Part model, mm, in its own coordinate system. A direction names the side the tool comes from. Round coordinates to 2 decimals unless told otherwise and drop trailing zeros. Loops run counter-clockwise (first coordinate to the right, second up) from the corner with the lowest first, then second, coordinate; pieces in that order, holes last.
(1) Tool access for faces 4 (the face through (21.977, 25.266, 252.144)), 5 (the face through (0, 0, 252)): list every direction of +Z, -Z, +X, -X, +Y, -Y with a clear straight run to the whole face (end or side of a thin tool).
(2) Flat gauge pins, fed straight in: pin 1 (6 mm diameter, centred on x = 4.5, y = 12.5, fed in from +Z); pin 2 (1.5 mm diameter, centred on y = 13, z = 176.5, fed in from +X); pin 3 (4 mm diameter, centred on y = -13.5, z = 102, fed in from -X); pin 4 (5 mm diameter, centred on x = 25, y = 20.5, fed in from +Z). Where does each tip first touch, or does it go through?
(3) Cut at A-A on x = 15.5. List the corners of the cut face in (y, z), then the cut area to 3 significant figures.
(4) Probe probe 1 along Y at (x, z) = (9.5, 61.5); probe 2 along X at (y, z) = (6.5, 422.5); probe 3 along Z at (x, y) = (13.5, 29). List the from-to ranges inside material, lowest first.
(5) Cut at B-B on z = 349. List the corners of the cut face in (x, y), then the cut area to 3 significant figures.
(6) Mould opens along Y. For faces 1 (the face through (21.977, -25.266, 252.144)), 2 (the face through (18, -32.5, 252)), 3 (the face through (18, 32.5, 252)) say: +Y half, -Y half, draft (parallel to the pull), parting line (faces both ways), or undercut.
(7) Cut at C-C on y = -11.5. List the corners of the cut face in (x, z), then the cut area to 3 significant figures.
Autodesk Inventor part; units mm, degrees
ref_plane "Начальная плоскость" through (0, 0, 32.5001) normal (0, 0, 1) x (1, 0, 0)
ref_plane "Конечная плоскость" through (0, 0, 478.0035) normal (0, 0, 1) x (1, 0, 0)
ref_plane "РабПлоскость8" through (169.2997, 3.5, 32.958) normal (0.0027, 0, -1) x (-1, 0, -0.0027)
ref_plane "Начальная плоскость" through (0, 0, 32.5001) normal (0, 0, 1) x (1, 0, 0)
ref_plane "Конечная плоскость" through (0, 0, 478.0035) normal (0, 0, 1) x (1, 0, 0)
sketch "Эскиз" plane through (0, 0, 0) normal (0, 0, 1) x (1, 0, 0)
  line L0 (36, -32.5) -> (0, -32.5)
  line L1 (36, -32.5) -> (36, -28.696)
  line L2 (33.6994, -26.2039) -> (9.9215, -24.3017)
  line L3 (4.4, -18.3208) -> (4.4, 18.3208)
  line L4 (33.6994, 26.2039) -> (9.9215, 24.3017)
  line L5 (36, 28.696) -> (36, 32.5)
  line L6 (0, 32.5) -> (36, 32.5)
  line L7 (0, -32.5) -> (0, 32.5)
  arc A0 (4.4, -18.3208) -> (9.9215, -24.3017) centre (10.4, -18.3208) ccw
  arc A1 (9.9215, 24.3017) -> (4.4, 18.3208) centre (10.4, 18.3208) ccw
  arc A2 (36, -28.696) -> (33.6994, -26.2039) centre (33.5, -28.696) ccw
  arc A3 (33.6994, 26.2039) -> (36, 28.696) centre (33.5, 28.696) ccw
  line L8 (0, 45.5) -> (0, -45.5) construction
  line L9 (-7.2974, 0) -> (43.7847, 0) construction
  point P0 (36, -26.388)
  point P1 (4.4, -23.86)
  point P2 (4.4, 23.86)
  point P3 (36, 26.388)
  dimension "d3" = 36
  dimension "d5" = 4.4
  dimension "d7" = 65
  dimension "d9" = 8.64
  dimension "d11" = 8.64
  dimension "d13" = 6.112
  dimension "d15" = 6.112
  dimension "d22" = 6
  dimension "d23" = 2.5
  dimension "d24" = 32.5
  dimension "d25" = 0
extrude "Тело" add sketch "Эскиз" along normal up to surface (445.5034 mm away) from surface at 32.5001
sketch "Sketch3" plane through (0, 0, 0) normal (0, 0, 1) x (1, 0, 0)
  line L0 (0, 0) -> (10, 0)
ref_plane "Work Plane7" through (0, 0, 0) normal (0, -1, 0) x (1, 0, 0)
sketch "Sketch4" plane through (0, 0, 0) normal (0, -1, 0) x (1, 0, 0)
  line L0 (-2, 32.5001) -> (12, 32.5001)
  line L1 (-2, 478.0035) -> (12, 478.0035)
  dimension "d29" = 445.5034
ref_plane "РабПлоскость8" through (169.2997, 3.5, 32.958) normal (0.0027, 0, -1) x (-1, 0, -0.0027)
split "Разделение1" plane through (169.2997, 3.5, 32.958) removes the side toward (0.0027, 0, -1)
ref_plane "РабПлоскость9" through (164.2926, -32.5, 478.3501) normal (-0.0027, 0, 1) x (1, 0, 0.0027)
split "Разделение2" plane through (164.2926, -32.5, 478.3501) removes the side toward (-0.0027, 0, 1)
equation "\"d3\" = b"
equation "\"d7\" = ParH"
equation "\"d22\" = R"
equation "\"d23\" = R1"
equation "\"d24\" = 0.5 * d7"
equation "\"d16\" = G_L"
equation "\"R1\" = 2.5"
equation "\"R\" = 6"
equation "\"t1\" = 4.4"
equation "\"t2\" = 7.2"
equation "\"ParH\" = 65"
equation "\"b\" = 36"
equation "\"msp_x1\" = 0.04 * b"
equation "\"msp_x2\" = -0.08 * t1 + 0.04 * b"
equation "\"G_L\" = d29"
equation "\"ex\" = 0"
equation "\"G_OFFSET_START\" = -32.50012"
equation "\"G_OFFSET_END\" = -35.90288"
equation "\"d26\" = -G_OFFSET_START"
equation "\"d27\" = G_OFFSET_END + B_L"
equation "\"B_L\" = 513.90637"
properties part number "Швеллер 6.5U-445,5 ГОСТ 8240-97" material "Сталь, мягкая"
Final values:
1. face 4: +Z, -Z, +X
1. face 5: +Z, -Z, -X, +Y, -Y
2. pin 1: stops at z = 477.92
2. pin 2: stops at x = 4.4
2. pin 3: stops at x = 0
2. pin 4: passes through
3. outline: (-32.5, 32.54) - (-24.75, 32.54) - (-24.75, 477.95) - (-32.5, 477.95) - close; (24.75, 32.54) - (32.5, 32.54) - (32.5, 477.95) - (24.75, 477.95) - close
3. area: 6,910 mm2
4. probe 1: y = -32.5 to -24.25, 24.25 to 32.5
4. probe 2: x = 0 to 4.4
4. probe 3: z = 32.54 to 477.94
5. outline: (0, -32.5) - (36, -32.5) - (36, -28.7) arc R2.5 ccw to (33.7, -26.2) - (9.92, -24.3) arc R6 cw to (4.4, -18.32) - (4.4, 18.32) arc R6 cw to (9.92, 24.3) - (33.7, 26.2) arc R2.5 ccw to (36, 28.7) - (36, 32.5) - (0, 32.5) - close
5. area: 763 mm2
6. face 1: undercut
6. face 2: -Y half
6. face 3: +Y half
7. outline: (0, 32.5) - (4.4, 32.51) - (4.4, 477.92) - (0, 477.91) - close
7. area: 1,960 mm2
